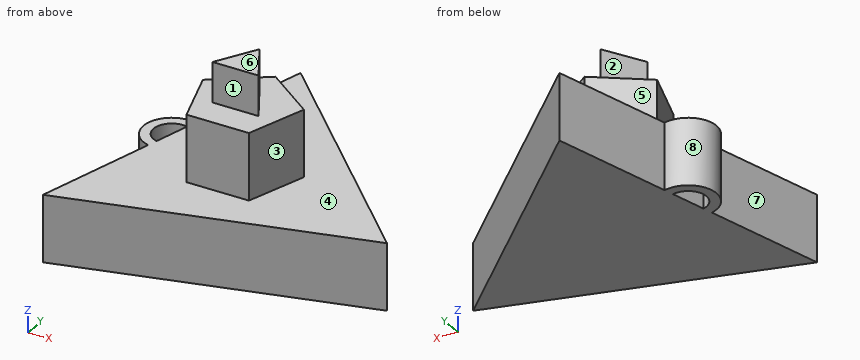
from build123d import *

# Parameters (mm, degrees)
F1_DEPTH = 6.35
F3_DEPTH = 6.35
F5_DEPTH = 3.81
F6_R     = 2.694583
F6_R_2   = 1.7341
F7_DEPTH = 6.35


with BuildPart() as f1:
    # F0 (on Top) → F1 (new body)
    with BuildSketch(Plane.XY):
        Polygon((16.356344, -4.382671), (-4.382668, 16.356344), (-11.973676, -11.973674), align=None)
    extrude(amount=F1_DEPTH)

    # F2 (on face) → F3 (join)
    with BuildSketch(Plane.XY.offset(6.35)):
        Polygon((-2.985949, -4.109806), (2.985949, -4.109806), (4.831367, 1.569806), (0, 5.08), (-4.831367, 1.569806), align=None)
    extrude(amount=F3_DEPTH)

    # F4 (on face) → F5 (join)
    with BuildSketch(Plane.XY.offset(12.7)):
        Polygon((-2.199705, -1.27), (2.199705, -1.27), (0, 2.54), align=None)
    extrude(amount=F5_DEPTH)

    # F6 (on face) → F7 (join)
    with BuildSketch(Plane.XY.offset(6.35)):
        with Locations((-8.178172, 2.191335)):
            Circle(F6_R)
        with Locations((-8.178172, 2.191335)):
            Circle(F6_R_2, mode=Mode.SUBTRACT)
    extrude(amount=-F7_DEPTH)


solid = f1.part
Can you work these out from the model? Positions are in its coordinate system, mm. Face numbers are marked on the shaded views. A direction names the side the tool comes from. Round coordinates to 2 decimals unless told otherwise and drop trailing zeros. Order: outer loops, then holes, each group sorted by start corner. A loop starts at its lowest first (then second) coordinate and runs counter-clockwise, first axis right, second up. Notation, with made-up numbers: (-16.75, 7.25) - (12.25, 7.25) arc R14 cw to (12.25, 25.25) - close; hole circle Ø7 at (-34.75, 26). An arc over 180 degrees is marked (long way). Answer in a Markdown table with one row per item.
(1) Suppose I cut it at B-B, the plane y = 1. Please give me the cut outline in (x, z).
From the geometry:
| item | result |
|---|---|
| outline | (-10.6, 0) - (-9.44, 0) - (-9.44, 6.35) - (-10.6, 6.35) - close; (-8.5, 0) - (10.97, 0) - (10.97, 6.35) - (4.65, 6.35) - (4.65, 12.7) - (0.89, 12.7) - (0.89, 16.51) - (-0.89, 16.51) - (-0.89, 12.7) - (-4.65, 12.7) - (-4.65, 6.35) - (-8.5, 6.35) - close |
(2) Suppose I cut it at A-A, the plane z = 2.75. Please give me the cut outline in (x, y).
From the geometry:
| item | result |
|---|---|
| outline | (-11.97, -11.97) - (16.36, -4.38) - (-4.38, 16.36) - (-7.48, 4.79) arc R2.69 ccw to (-8.88, -0.41) - close; hole (-8.63, 0.52) - (-7.73, 3.87) arc R1.73 ccw to start |
(3) Suppose I cut it at D-D, the plane x = 0.5. Please give me the cut outline in (y, z).
From the geometry:
| item | result |
|---|---|
| outline | (-8.63, 0) - (11.47, 0) - (11.47, 6.35) - (4.72, 6.35) - (4.72, 12.7) - (1.67, 12.7) - (1.67, 16.51) - (-1.27, 16.51) - (-1.27, 12.7) - (-4.11, 12.7) - (-4.11, 6.35) - (-8.63, 6.35) - close |
(4) If we mould it in two halves opening along Y, with no side actions, what happens to the marked faces 5, 6, 7 and 8? For each: released by +Y, released by -Y, zero draft, split by the parting line, or undercut.
From the geometry:
| item | result |
|---|---|
| face 5 | released by +Y |
| face 6 | zero draft |
| face 7 | undercut |
| face 8 | undercut |
(5) Suppose I cut it at C-C, the plane z = 9.5. Please give me the cut outline in (x, y).
From the geometry:
| item | result |
|---|---|
| outline | (-4.83, 1.57) - (-2.99, -4.11) - (2.99, -4.11) - (4.83, 1.57) - (0, 5.08) - close |
(6) For P1, Ø5, axis at x = 8, z = 13.5, coming from the -Y side; P2, Ø1.8, axis at x = 0.5, z = 8, coming from the -Y side; P3, Ø6, axis at x = 7, z = 4, coming from the -Y side; P4, Ø1.5, axis at y = 3, z = 14.5, coming from the -X side, each with a flat end and sliding along its axis, tell me the tip position at first contact or that it passes through.
From the geometry:
| item | result |
|---|---|
| P1 | passes through |
| P2 | stops at y = -4.11 |
| P3 | stops at y = -7.69 |
| P4 | stops at x = -0.17 |
(7) Please list where these lines run through material, in increasing order: L1, parallel to Z at x = -1, y = 2.75; L2, parallel to Z at x = 13, y = -5; L3, parallel to Y at x = -0.5, z = 13.25. Write a range as from..to.
From the geometry:
| item | result |
|---|---|
| L1 | z = 0..12.7 |
| L2 | z = 0..6.35 |
| L3 | y = -1.27..1.67 |
(8) Which directions (+Z, -Z, +X, -X, +Y, -Y) give clear straight access to the entire face, cutting with the end or side of a thin tool? Please do the marked faces 1, 2, 3 and 4.
From the geometry:
| item | result |
|---|---|
| face 1 | +Z, +X, -X, -Y |
| face 2 | +Z, -X, +Y |
| face 3 | +Z, +X, -Y |
| face 4 | +Z |
